Design review of the part built by this model. Coordinates are the model's own, in mm. A direction names the side the tool comes from. Coordinates: 2 decimals unless noted, no trailing zeros. Write each loop counter-clockwise with the first axis right and the second up, starting at its lowest first coordinate (ties: lowest second). Pieces come first, ordered by that corner, then holes. Notation, with made-up numbers: (-35.75, 46) -> (-28.75, 46) arc R31 ccw to (-28.75, 73) -> close; hole circle Ø4 at (13, 38). An arc over 180 degrees is marked (long way). One line per question, with ' | ' between items. Start each with the question number.
Q1. Add section D-D on x = -14.5. State the section outline as (y, z) points, and give its area (3 significant figures).
Q2. Add section A-A on x = 0. State the section outline as (y, z) points, and give its area (4 significant figures).
Q3. For faces 1 (the flat face through (-30.841, 10.888, -0.105)), 2 (the flat face through (-3, 32.6, -0.1)), 3 (the flat face through (-8.3, -31.63, -0.11)), 4 (the flat face through (30.901, 10.946, -0.105)), list the 3-axis set-ups (+Z, -Z, +X, -X, +Y, -Y) from which the entire face can be reached by the end or side of a thin tool; tool diameter is ignored.
Q4. Wall thickness on probe 1 along Y at (x, z) = (0, 4); probe 2 along X at (y, z) = (-30, 0.75); probe 3 along X at (y, z) = (-30.5, -3): over which ranges is each line inside the solid? List them lowest first.
Q5. Add section C-C on y = -14.5. State the section outline as (x, z) points.
Q6. Add section B-B on y = -5. State the section outline as (x, z) points.
Q7. For P1, Ø1.5, axis at y = 26.5, z = 4, coming from the -X side; P2, Ø8, axis at x = -17.5, z = -3.5, coming from the -Y side; P3, Ø1.2, axis at y = 10.5, z = -1, coming from the +X side, all flat-tipped, find the tip position at first contact; note any pin that passes through.
from build123d import *

# Parameters (mm, degrees)
SKETCH1_R           = 35.5
BOSS_EXTRUDE1_DEPTH = 7.5
CUT_EXTRUDE2_START  = -15
CUT_EXTRUDE2_DEPTH  = 15


# Read off the part's stored shape, not the designer's step: Cut-Extrude2
with BuildPart() as part:
    # Sketch1 → Boss-Extrude1 (new, symmetric)
    with BuildSketch(Plane.XY):
        Circle(SKETCH1_R)
        with BuildLine():
            Line((-2.5, 12), (2.5, 12))
            Line((2.5, 12), (2.5, 9.682458366))
            ThreePointArc((2.5, 9.682458366), (0, -10), (-2.5, 9.682458366))
            Line((-2.5, 9.682458366), (-2.5, 12))
        make_face(mode=Mode.SUBTRACT)
    extrude(amount=BOSS_EXTRUDE1_DEPTH, both=True)

    # Cut-Extrude2 outline → Cut-Extrude2 (cut)
    with BuildSketch(Plane.XY.offset(7.5).offset(CUT_EXTRUDE2_START)):
        with BuildLine():
            Line((-15.698524782, 31.84032537), (-11.159709939, 27.887468047))
            Line((-11.159709939, 27.887468047), (-8.322258214, 28.861566455))
            Line((-8.322258214, 28.861566455), (-7.168390776, 34.768724073))
            ThreePointArc((-7.168390776, 34.768724073), (-11.526831157, 33.57651208), (-15.698524782, 31.84032537))
        make_face()
        with BuildLine():
            Line((-17.242670617, 24.595534351), (-18.069373842, 30.557286021))
            ThreePointArc((-18.069373842, 30.557286021), (-21.8045513, 28.014488084), (-25.186472155, 25.017826053))
            Line((-25.186472155, 25.017826053), (-19.610092145, 22.752896213))
            Line((-19.610092145, 22.752896213), (-17.242670617, 24.595534351))
        make_face()
        with BuildLine():
            ThreePointArc((4.509398661, 35.21243138), (0, 35.5), (-4.509398661, 35.21243138))
            Line((-4.509398661, 35.21243138), (-1.5, 30))
            Line((-1.5, 30), (1.5, 30))
            Line((1.5, 30), (4.509398661, 35.21243138))
        make_face()
        with BuildLine():
            Line((-24.294572111, 17.664194461), (-27.012259878, 23.034491882))
            ThreePointArc((-27.012259878, 23.034491882), (-29.719409978, 19.416659613), (-31.945074461, 15.484257091))
            Line((-31.945074461, 15.484257091), (-25.935416585, 15.152695026))
            Line((-25.935416585, 15.152695026), (-24.294572111, 17.664194461))
        make_face()
        with BuildLine():
            ThreePointArc((15.698524782, 31.84032537), (11.526831157, 33.57651208), (7.168390776, 34.768724073))
            Line((7.168390776, 34.768724073), (8.322258214, 28.861566455))
            Line((8.322258214, 28.861566455), (11.159709939, 27.887468047))
            Line((11.159709939, 27.887468047), (15.698524782, 31.84032537))
        make_face()
        with BuildLine():
            Line((-28.713779747, 8.818665013), (-33.027948418, 13.015553132))
            ThreePointArc((-33.027948418, 13.015553132), (-34.413709441, 8.714734794), (-35.241932271, 4.27272861))
            Line((-35.241932271, 4.27272861), (-29.450236209, 5.910464215))
            Line((-29.450236209, 5.910464215), (-28.713779747, 8.818665013))
        make_face()
        with BuildLine():
            ThreePointArc((25.186472155, 25.017826053), (21.8045513, 28.014488084), (18.069373842, 30.557286021))
            Line((18.069373842, 30.557286021), (17.242670617, 24.595534351))
            Line((17.242670617, 24.595534351), (19.610092145, 22.752896213))
            Line((19.610092145, 22.752896213), (25.186472155, 25.017826053))
        make_face()
        with BuildLine():
            Line((-30.021403808, -0.982503625), (-35.464546265, 1.586177242))
            ThreePointArc((-35.464546265, 1.586177242), (-35.378749502, -2.931566764), (-34.719779885, -7.401816314))
            Line((-34.719779885, -7.401816314), (-29.773665772, -3.972257104))
            Line((-29.773665772, -3.972257104), (-30.021403808, -0.982503625))
        make_face()
        with BuildLine():
            ThreePointArc((31.945074461, 15.484257091), (29.719409978, 19.416659613), (27.012259878, 23.034491882))
            Line((27.012259878, 23.034491882), (24.294572111, 17.664194461))
            Line((24.294572111, 17.664194461), (25.935416585, 15.152695026))
            Line((25.935416585, 15.152695026), (31.945074461, 15.484257091))
        make_face()
        with BuildLine():
            Line((-28.075742937, -10.67720275), (-34.058010235, -10.015085564))
            ThreePointArc((-34.058010235, -10.015085564), (-32.509953096, -14.260187575), (-30.435200615, -18.274259589))
            Line((-30.435200615, -18.274259589), (-26.870656663, -13.42452273))
            Line((-26.870656663, -13.42452273), (-28.075742937, -10.67720275))
        make_face()
        with BuildLine():
            ThreePointArc((35.241932271, 4.27272861), (34.413709441, 8.714734794), (33.027948418, 13.015553132))
            Line((33.027948418, 13.015553132), (28.713779747, 8.818665013))
            Line((28.713779747, 8.818665013), (29.450236209, 5.910464215))
            Line((29.450236209, 5.910464215), (35.241932271, 4.27272861))
        make_face()
        with BuildLine():
            Line((-23.087639678, -19.214861283), (-28.960760331, -20.531058449))
            ThreePointArc((-28.960760331, -20.531058449), (-26.118198829, -24.043495793), (-22.852495108, -27.166403283))
            Line((-22.852495108, -27.166403283), (-21.055794963, -21.422033015))
            Line((-21.055794963, -21.422033015), (-23.087639678, -19.214861283))
        make_face()
        with BuildLine():
            ThreePointArc((34.719779885, -7.401816314), (35.378749502, -2.931566764), (35.464546265, 1.586177242))
            Line((35.464546265, 1.586177242), (30.021403808, -0.982503625))
            Line((30.021403808, -0.982503625), (29.773665772, -3.972257104))
            Line((29.773665772, -3.972257104), (34.719779885, -7.401816314))
        make_face()
        with BuildLine():
            Line((-15.597632418, -25.670291447), (-20.725162674, -28.822172579))
            ThreePointArc((-20.725162674, -28.822172579), (-16.896132453, -31.221318168), (-12.793367162, -33.114645652))
            Line((-12.793367162, -33.114645652), (-12.959211164, -27.098133626))
            Line((-12.959211164, -27.098133626), (-15.597632418, -25.670291447))
        make_face()
        with BuildLine():
            ThreePointArc((30.435200615, -18.274259589), (32.509953096, -14.260187575), (34.058010235, -10.015085564))
            Line((34.058010235, -10.015085564), (28.075742937, -10.67720275))
            Line((28.075742937, -10.67720275), (26.870656663, -13.42452273))
            Line((26.870656663, -13.42452273), (30.435200615, -18.274259589))
        make_face()
        with BuildLine():
            Line((-6.417379664, -29.343947217), (-10.243672056, -33.989957087))
            ThreePointArc((-10.243672056, -33.989957087), (-5.843107955, -35.015826271), (-1.347879375, -35.474402337))
            Line((-1.347879375, -35.474402337), (-3.458295753, -29.837730988))
            Line((-3.458295753, -29.837730988), (-6.417379664, -29.343947217))
        make_face()
        with BuildLine():
            ThreePointArc((22.852495108, -27.166403283), (26.118198829, -24.043495793), (28.960760331, -20.531058449))
            Line((28.960760331, -20.531058449), (23.087639678, -19.214861283))
            Line((23.087639678, -19.214861283), (21.055794963, -21.422033015))
            Line((21.055794963, -21.422033015), (22.852495108, -27.166403283))
        make_face()
        with BuildLine():
            Line((3.458295753, -29.837730988), (1.347879375, -35.474402337))
            ThreePointArc((1.347879375, -35.474402337), (5.843107955, -35.015826271), (10.243672056, -33.989957087))
            Line((10.243672056, -33.989957087), (6.417379664, -29.343947217))
            Line((6.417379664, -29.343947217), (3.458295753, -29.837730988))
        make_face()
        with BuildLine():
            ThreePointArc((12.793367162, -33.114645652), (16.896132453, -31.221318168), (20.725162674, -28.822172579))
            Line((20.725162674, -28.822172579), (15.597632418, -25.670291447))
            Line((15.597632418, -25.670291447), (12.959211164, -27.098133626))
            Line((12.959211164, -27.098133626), (12.793367162, -33.114645652))
        make_face()
    extrude(amount=CUT_EXTRUDE2_DEPTH, mode=Mode.SUBTRACT)


solid = part.part
Output values:
1) outline: (-26.26, -7.5) -> (30.8, -7.5) -> (30.8, 7.5) -> (-26.26, 7.5) -> close | area: 856 mm2
2) outline: (-35.5, -7.5) -> (-10, -7.5) -> (-10, 7.5) -> (-35.5, 7.5) -> close; (12, -7.5) -> (30, -7.5) -> (30, 7.5) -> (12, 7.5) -> close | area: 652.5 mm2
3) face 1: +Z, -Z, -X | face 2: +Z, -Z, +Y | face 3: +Z, -Z, -Y | face 4: +Z, -Z, +X
4) probe 1: y = -35.5 to -10, 12 to 30 | probe 2: x = -12.88 to -6.96, -3.4 to 3.4, 6.96 to 12.88 | probe 3: x = -12.87 to -7.37, -3.21 to 3.21, 7.37 to 12.87
5) outline: (-27.66, -7.5) -> (27.66, -7.5) -> (27.66, 7.5) -> (-27.66, 7.5) -> close
6) outline: (-31.26, -7.5) -> (-8.66, -7.5) -> (-8.66, 7.5) -> (-31.26, 7.5) -> close; (8.66, -7.5) -> (31.26, -7.5) -> (31.26, 7.5) -> (8.66, 7.5) -> close
7) P1: stops at x = -17.61 | P2: stops at y = -28.82 | P3: stops at x = 31.06
